Could you check a few things on this model? Use its own coordinates, in mm. A direction names the side the tool comes from. Give positions to 0.01 mm unless a question says otherwise; leave off trailing zeros. Loops run counter-clockwise (first coordinate to the right, second up) from the corner with the lowest first, then second, coordinate; pieces in that order, holes last. Notation, with made-up numbers: (29.25, -28) - (85.25, -28) arc R27 cw to (85.25, 6) - close; hole circle Ø3 at (89, 35). An arc over 180 degrees is marked (long way). Use CSV: the item, a comma, the result in double quotes.
from build123d import *

# Parameters (mm, degrees)
SKETCH_1_W          = 60
SKETCH_1_H          = 40
EXTRUDE_1_DEPTH     = 200
SKETCH_6_R          = 20
EXTRUDE_2_DEPTH     = 20
EXTRUDE_START       = -20
SKETCH_7_R          = 20
EXTRUDE_3_DEPTH     = 20
SKETCH_8_R          = 10
CUT_EXTRUDE_1_DEPTH = 211.297408448
SKETCH_9_R          = 20
CUT_EXTRUDE_2_DEPTH = 20


with BuildPart() as part:
    # 스케치1 → 보스-돌출1 (new body)
    with BuildSketch(Plane.XY):
        with Locations((20, 5)):
            Rectangle(SKETCH_1_W, SKETCH_1_H)
    extrude(amount=EXTRUDE_1_DEPTH)

    # 스케치6 → 보스-돌출2 (add)
    with BuildSketch(Plane(origin=(50, 0, 0), x_dir=(0, 0, -1), z_dir=(1, 0, 0))):
        with Locations((0, 5)):
            Circle(SKETCH_6_R)
    extrude_2 = extrude(amount=-EXTRUDE_2_DEPTH)

    # 스케치7 → 보스-돌출3 (add)
    with BuildSketch(Plane.ZY.offset(10).offset(EXTRUDE_START)):
        with Locations((0, 5)):
            Circle(SKETCH_7_R)
    extrude_3 = extrude(amount=EXTRUDE_3_DEPTH)

    # 스케치8 → 컷-돌출1 (cut, symmetric)
    with BuildSketch(Plane.ZY.offset(10)):
        with Locations((0, 5)):
            Circle(SKETCH_8_R)
    cut_extrude_1 = extrude(amount=CUT_EXTRUDE_1_DEPTH, both=True, mode=Mode.SUBTRACT)

    # 대칭 복사1: 보스-돌출2, 보스-돌출3, 컷-돌출1 across plane
    add(extrude_2.mirror(Plane.XY.offset(100)))
    add(extrude_3.mirror(Plane.XY.offset(100)))
    add(cut_extrude_1.mirror(Plane.XY.offset(100)), mode=Mode.SUBTRACT)

    # 스케치9 → 컷-돌출2 (cut)
    with BuildSketch(Plane.ZY.offset(-30)):
        with Locations((0, 5)):
            Circle(SKETCH_9_R)
    extrude(amount=CUT_EXTRUDE_2_DEPTH, mode=Mode.SUBTRACT)


solid = part.part
1) Suppose I cut it at C-C (z = 4.5). Please give me the cut outline in (x, y).
Answer below:
outline,"(-10, -15) - (50, -15) - (50, -3.93) - (30, -3.93) - (30, -14.49) - (10, -14.49) - (10, -3.93) - (-10, -3.93) - close; (-10, 13.93) - (10, 13.93) - (10, 24.49) - (30, 24.49) - (30, 13.93) - (50, 13.93) - (50, 25) - (-10, 25) - close"
2) Suppose I cut it at B-B (x = 7). Please give me the cut outline in (y, z), plus the area to 3 significant figures.
Answer below:
outline,"(-15, 0) arc R20 ccw to (25, 0) - (25, 200) arc R20 ccw to (-15, 200) - close; hole circle Ø20 at (5, 0); hole circle Ø20 at (5, 200)"
area,"8,630 mm2"
3) I'm going to push flat-ended pins straight in: P1, Ø11, axis at x = 18, y = -8.5, coming from the +Z side; P2, Ø2, axis at x = 30.5, y = 7, coming from the +Z side (3 decimals); P3, Ø18, axis at y = 5, z = 0, coming from the -X side; P4, Ø4, axis at x = 34.5, y = 10.5, coming from the +Z side. Where does each tip first touch, or does it pass through?
Answer below:
P1,"stops at z = 200"
P2,"stops at z = 219.975"
P3,"passes through"
P4,"stops at z = 219.69"
4) I need wall thicknesses on line 1 along Z through (x, y) = (6.5, 5); line 2 along X through (y, z) = (1, 209.5); line 3 along Y through (x, z) = (46, 1). Which ranges of each line are inside material? Lowest first, please.
Answer below:
line 1,"z = -20 to -10, 10 to 190, 210 to 220"
line 2,"x = -10 to 10, 30 to 50"
line 3,"y = -15 to -4.95, 14.95 to 25"
5) Which directions (+Z, -Z, +X, -X, +Y, -Y) give clear straight access to the entire face, cutting with the end or side of a thin tool? Please do faces 1 (the cylindrical face through (0, 5, -20)), 2 (the cylindrical face through (20, 5, 20)), 3 (the flat face through (20, 20, 200)).
Answer below:
face 1,"-Z, +X, -X"
face 2,"-Z"
face 3,"+Z, +Y, -Y"
6) Suppose I cut it at D-D (x = 16.5). Please give me the cut outline in (y, z).
Answer below:
outline,"(-15, 0) arc R20 cw to (25, 0) - (25, 200) - (15, 200) arc R10 cw to (-5, 200) - (-15, 200) - close"
7) Suppose I cut it at A-A (y = 5). Please give me the cut outline in (x, z), plus the area to 3 significant figures.
Answer below:
outline,"(-10, -20) - (10, -20) - (10, -10) - (-10, -10) - close; (-10, 10) - (10, 10) - (10, 20) - (30, 20) - (30, 10) - (50, 10) - (50, 190) - (-10, 190) - close; (-10, 210) - (10, 210) - (10, 220) - (-10, 220) - close; (30, -20) - (50, -20) - (50, -10) - (30, -10) - close; (30, 210) - (50, 210) - (50, 220) - (30, 220) - close"
area,"11,400 mm2"
8) We'd pull the mould along Z, two halves only. Please class faces 4 (the flat face through (20, -10, 200)), 5 (the flat face through (10, 14, -5)), 6 (the cylindrical face through (39.86, 14.915, -1.302)), 7 (the cylindrical face through (-0.14, 14.915, -1.302)): +Z half, -Z half, draft (parallel to the pull), parting line (faces both ways), or undercut.
Answer below:
face 4,"+Z half"
face 5,"draft"
face 6,"undercut"
face 7,"undercut"
